For this review, use the dimensioned drawing (mm, ordinates from the lowest corner) and the shaded views. A direction names the side the tool comes from. Coordinates: 2 decimals unless noted, no trailing zeros. Order: outer loops, then holes, each group sorted by start corner. A loop starts at its lowest first (then second) coordinate and runs counter-clockwise, first axis right, second up. Notation, with made-up numbers: M 8.25,26 L 56.25,26 A18 ccw 56.25,60 Z; hole C 10,-25.5 d10. An arc over 180 degrees is marked long. Answer as CSV lines item,"result". Start each with the question number.
Q1. Machinability: for the marked faces 1 and 2, which of the approach directions +Z, -Z, +X, -X, +Y, -Y give a long, thin tool a straight path to every point of the face, cutting with its end or side? Answer none if there is none.
Q2. The part is to be moulded in two halves that separate along X. For the marked faces 3, 4 and 5, say which applies: +X half, -X half, draft (parallel to the pull), parting line (faces both ways), or undercut.
Q3. Consider section B-B on z = 27. Write out the cut boundary in (x, y).
Q4. Wall thickness on L1, parallel to X at y = 30, z = 33.5; L2, parallel to Z at x = 19.5, y = 25.5; L3, parallel to Z at x = 46, y = 8.5 (1 decimal): over which ranges is each line inside the solid? List them lowest first. Write a range as [from, to].
Q5. For P1, Ø8, axis at x = 9.5, z = 28.5, coming from the -Y side; P2, Ø6, axis at x = 27, y = 25, coming from the +Z side; P3, Ø8, axis at x = 39.5, y = 16, coming from the +Z side, all flat-tipped, find the tip position at first contact; note any pin that passes through.
Q6. Consider section D-D on x = 39.5. Write out the cut boundary in (y, z).
Q7. Consider section C-C on y = 29.5. Write out the cut boundary in (x, z), and give its area (3 significant figures).
Q8. Consider section A-A on x = 18. Write out the cut boundary in (y, z).
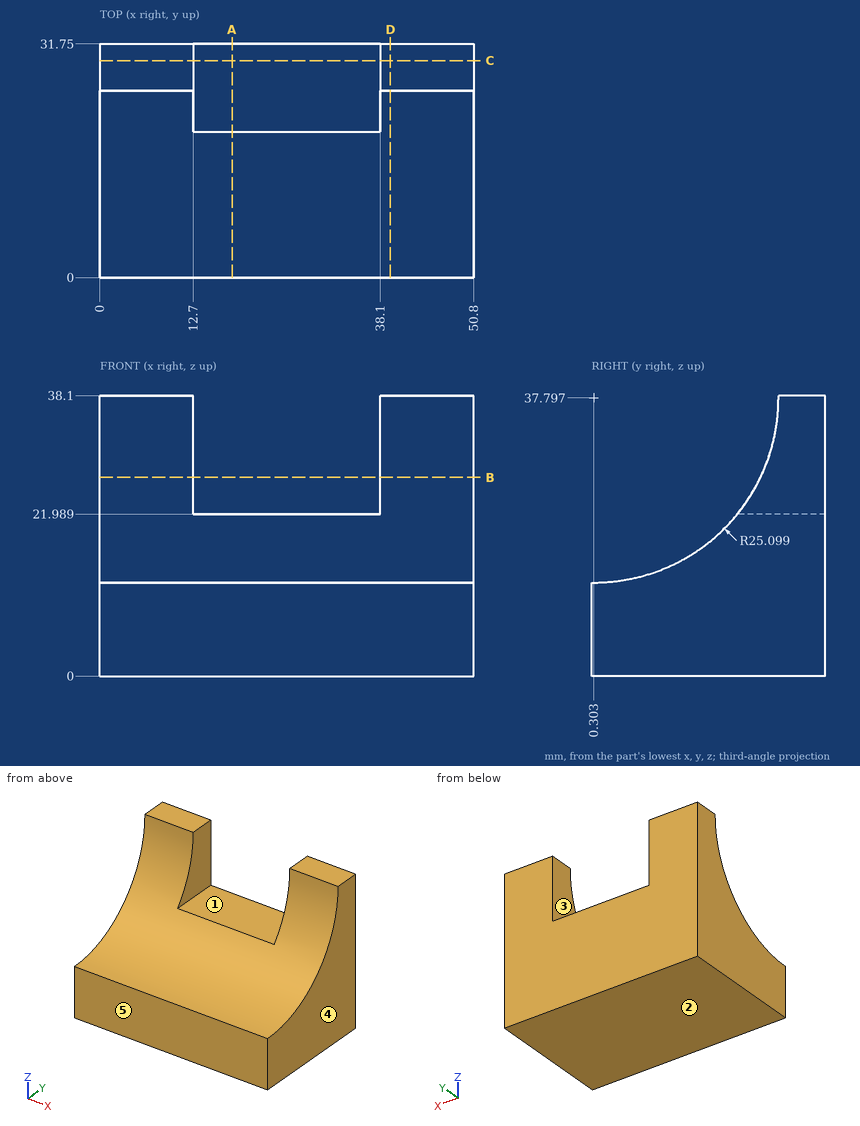
Evaluation:
1,face 1,"+Z, +Y, -Y"
1,face 2,"-Z, +X, -X, +Y, -Y"
2,face 3,"undercut"
2,face 4,"+X half"
2,face 5,"draft"
3,outline,"M 0,22.96 L 12.7,22.96 L 12.7,31.75 L 0,31.75 Z; M 38.1,22.96 L 50.8,22.96 L 50.8,31.75 L 38.1,31.75 Z"
4,L1,"x = [0, 12.7], [38.1, 50.8]"
4,L2,"z = [0, 21.99]"
4,L3,"z = [0, 14.1]"
5,P1,"stops at y = 21.59"
5,P2,"stops at z = 21.99"
5,P3,"stops at z = 22.24"
6,outline,"M 0,0 L 31.75,0 L 31.75,38.1 L 25.4,38.1 A25.1 cw 0,12.7 Z"
7,outline,"M 0,0 L 50.8,0 L 50.8,38.1 L 38.1,38.1 L 38.1,21.99 L 12.7,21.99 L 12.7,38.1 L 0,38.1 Z"
7,area,"1,530 mm²"
8,outline,"M 0,0 L 31.75,0 L 31.75,21.99 L 19.8,21.99 A25.1 cw 0,12.7 Z"
